```python
from build123d import *

# Parameters (mm, degrees)
EXTRUDE_1_DEPTH     = 295
SKETCH_2_R          = 1
CUT_EXTRUDE_1_DEPTH = 10
CHAMFER_1_SIZE      = 0.5
SKETCH_3_R          = 2.383304988
CUT_EXTRUDE_2_DEPTH = 1


with BuildPart() as part:
    # 草图1 → 凸台-拉伸1 (new body)
    with BuildSketch(Plane(origin=(0, 0, 0), x_dir=(1, 0, 0), z_dir=(0, 1, 0))):
        Polygon((-3.5, 0.4), (-3.5, -2.4), (3.5, -2.4), (3.5, 0.4), (2.5, 0.4), (2.5, 1.4), (3.5, 1.4), (3.5, 2.4), (-3.5, 2.4), (-3.5, 1.4), (-2.5, 1.4), (-2.5, 0.4), align=None)
    extrude(amount=EXTRUDE_1_DEPTH)

    # 草图2 → 切除-拉伸1 (cut)
    with BuildSketch(Plane(origin=(0, 0, -2.4), x_dir=(-1, 0, 0), z_dir=(0, 0, -1))):
        with Locations((0, 5)):
            Circle(SKETCH_2_R)
        with Locations((0, 20)):
            Circle(SKETCH_2_R)
        with Locations((0, 35)):
            Circle(SKETCH_2_R)
        with Locations((0, 50)):
            Circle(SKETCH_2_R)
        with Locations((0, 65)):
            Circle(SKETCH_2_R)
        with Locations((0, 80)):
            Circle(SKETCH_2_R)
        with Locations((0, 95)):
            Circle(SKETCH_2_R)
        with Locations((0, 110)):
            Circle(SKETCH_2_R)
        with Locations((0, 125)):
            Circle(SKETCH_2_R)
        with Locations((0, 140)):
            Circle(SKETCH_2_R)
        with Locations((0, 155)):
            Circle(SKETCH_2_R)
        with Locations((0, 170)):
            Circle(SKETCH_2_R)
        with Locations((0, 185)):
            Circle(SKETCH_2_R)
        with Locations((0, 200)):
            Circle(SKETCH_2_R)
        with Locations((0, 215)):
            Circle(SKETCH_2_R)
        with Locations((0, 230)):
            Circle(SKETCH_2_R)
        with Locations((0, 245)):
            Circle(SKETCH_2_R)
        with Locations((0, 260)):
            Circle(SKETCH_2_R)
        with Locations((0, 275)):
            Circle(SKETCH_2_R)
        with Locations((0, 290)):
            Circle(SKETCH_2_R)
    extrude(amount=-CUT_EXTRUDE_1_DEPTH, mode=Mode.SUBTRACT)

    # 倒角1
    chamfer_1_edges = [part.edges().sort_by_distance(p)[0] for p in [
        (-3.5, 147.5, -2.4),
        (3.5, 147.5, -2.4),
        (3.5, 147.5, 2.4),
        (-3.5, 147.5, 2.4),
    ]]
    chamfer(chamfer_1_edges, length=CHAMFER_1_SIZE)

    # 草图3 → 切除-拉伸2 (cut)
    with BuildSketch(Plane(origin=(0, 0, -2.4), x_dir=(-1, 0, 0), z_dir=(0, 0, -1))):
        with Locations((0, 5)):
            Circle(SKETCH_3_R)
        with Locations((0, 20)):
            Circle(SKETCH_3_R)
        with Locations((0, 35)):
            Circle(SKETCH_3_R)
        with Locations((0, 50)):
            Circle(SKETCH_3_R)
        with Locations((0, 65)):
            Circle(SKETCH_3_R)
        with Locations((0, 80)):
            Circle(SKETCH_3_R)
        with Locations((0, 95)):
            Circle(SKETCH_3_R)
        with Locations((0, 110)):
            Circle(SKETCH_3_R)
        with Locations((0, 125)):
            Circle(SKETCH_3_R)
        with Locations((0, 140)):
            Circle(SKETCH_3_R)
        with Locations((0, 155)):
            Circle(SKETCH_3_R)
        with Locations((0, 170)):
            Circle(SKETCH_3_R)
        with Locations((0, 185)):
            Circle(SKETCH_3_R)
        with Locations((0, 200)):
            Circle(SKETCH_3_R)
        with Locations((0, 215)):
            Circle(SKETCH_3_R)
        with Locations((0, 230)):
            Circle(SKETCH_3_R)
        with Locations((0, 245)):
            Circle(SKETCH_3_R)
        with Locations((0, 260)):
            Circle(SKETCH_3_R)
        with Locations((0, 275)):
            Circle(SKETCH_3_R)
        with Locations((0, 290)):
            Circle(SKETCH_3_R)
    extrude(amount=-CUT_EXTRUDE_2_DEPTH, mode=Mode.SUBTRACT)


solid = part.part
```
Model file for the job. Use its own axes, mm. A direction names the side the tool comes from. Give positions to 0.01 mm unless a question says otherwise; leave off trailing zeros. Write each loop counter-clockwise with the first axis right and the second up, starting at its lowest first coordinate (ties: lowest second). Pieces come first, ordered by that corner, then holes. Notation, with made-up numbers: M -17.5,24 L 39.5,24 A13 ccw 39.5,34 Z; hole C -23.5,1.25 d3. An arc over 180 degrees is marked long. Use a Markdown table: item, result.
1) Pin check, flat tip, straight feed: pin 1 (3 mm diameter, centred on x = 0, y = 170, fed in from -Z). Stop position of the tip, or through.
Responses:
| item | result |
|---|---|
| pin 1 | stops at z = -1.4 |
2) Tool access for faces 1 (the cylindrical face through (0.517, 257.673, -1.907)), 2 (the flat face through (0, 295, 0)): list every direction of +Z, -Z, +X, -X, +Y, -Y with a clear straight run to the whole face (end or side of a thin tool).
Responses:
| item | result |
|---|---|
| face 1 | -Z |
| face 2 | +Z, -Z, +X, -X, +Y |
3) Cut at A-A (y = 221.5). List the corners of the cut face in (x, z).
Responses:
| item | result |
|---|---|
| outline | M -3.5,-1.9 L -3,-2.4 L 3,-2.4 L 3.5,-1.9 L 3.5,-1.4 L 2.5,-1.4 L 2.5,-0.4 L 3.5,-0.4 L 3.5,1.9 L 3,2.4 L -3,2.4 L -3.5,1.9 L -3.5,-0.4 L -2.5,-0.4 L -2.5,-1.4 L -3.5,-1.4 Z |
4) Pull direction X, two halves, no side cores. Call faces 3 (the flat face through (0, 145, 2.4)), 4 (the cylindrical face through (-1.1, 182.886, -1.907)): +X half, -X half, draft (parallel to the pull), parting line (faces both ways), or undercut.
Responses:
| item | result |
|---|---|
| face 3 | draft |
| face 4 | undercut |
5) Drill centre lines: line 1 (X direction, y = 185, z = -1.8); line 2 (Z direction, x = 3, y = 183); line 3 (X direction, y = 185, z = -0.6). Where is each one in solid material? Low to high. Write a range as from..to.
Responses:
| item | result |
|---|---|
| line 1 | x = -3.5..-2.38, 2.38..3.5 |
| line 2 | z = -2.4..-1.4, -0.4..2.4 |
| line 3 | x = -2.5..-1, 1..2.5 |
6) Cut at B-B (z = 1.05). Give the number of separate pieces and of enclosed holes in the cut face, and give its area (3 significant figures).
Responses:
| item | result |
|---|---|
| separate pieces | 1 |
| enclosed holes | 20 |
| area | 2,000 mm2 |
